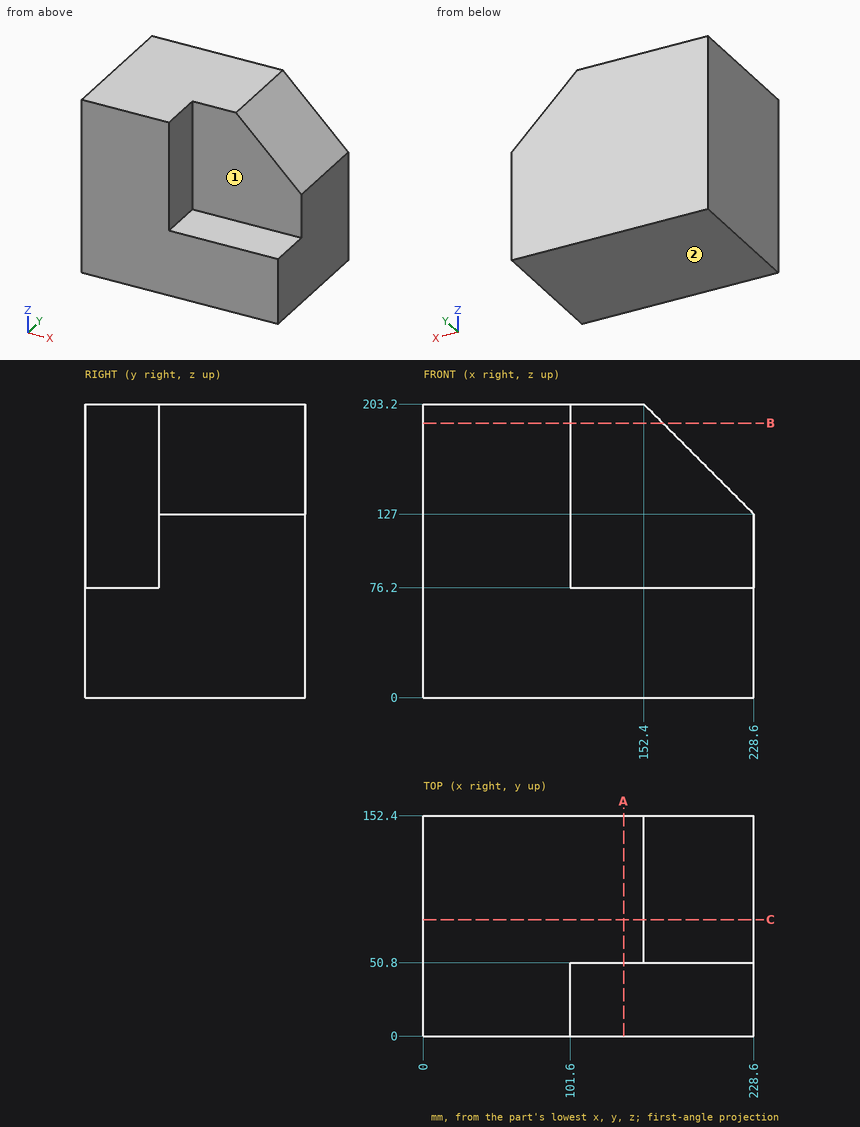
Source: three-view drawing plus pictorial views. Frame: mm from the lowest corner of the part. A direction names the side the tool comes from. Coordinates: 2 decimals unless noted, no trailing zeros. Order: outer loops, then holes, each group sorted by start corner. A loop starts at its lowest first (then second) coordinate and runs counter-clockwise, first axis right, second up. Notation, with made-up numbers: (39, 61.25) -> (70, 61.25) arc R22 ccw to (70, 70.25) -> close; hole circle Ø5 at (-23.75, 0.5). An arc over 180 degrees is marked (long way). Write item = value, one per line.
(1) Cut plane B-B on z = 190. Return loops of the section in (x, y), plus the area to 3 significant figures.
Solved:
outline = (0, 0) -> (101.6, 0) -> (101.6, 50.8) -> (165.6, 50.8) -> (165.6, 152.4) -> (0, 152.4) -> close
area = 22,000 mm²
(2) Line query: line 1 (Z direction, x = 190.5, y = 46); line 2 (Y direction, x = 163, z = 125); line 3 (X direction, y = 50, z = 114.5). Output: solid intervals per line, ascending.
Solved:
line_1 = 0 to 76.2
line_2 = 50.8 to 152.4
line_3 = 0 to 101.6
(3) Cut plane A-A on x = 138.5. Return loops of the section in (y, z), plus the area to 3 significant figures.
Solved:
outline = (0, 0) -> (152.4, 0) -> (152.4, 203.2) -> (50.8, 203.2) -> (50.8, 76.2) -> (0, 76.2) -> close
area = 24,500 mm²
(4) Access query for the marked faces 1 and 2. Directions: +Z, -Z, +X, -X, +Y, -Y. A direction counts if a zero-diameter tool reaches every point of the face in a straight line with its end or side. Return the directions, or none.
Solved:
face_1 = +Z, +X, -Y
face_2 = -Z, +X, -X, +Y, -Y
(5) Cut plane C-C on y = 80.5. Return loops of the section in (x, z).
Solved:
outline = (0, 0) -> (228.6, 0) -> (228.6, 127) -> (152.4, 203.2) -> (0, 203.2) -> close
(6) Pin query (flat end, axial travel): pin 1 Ø1 at (x, z) = (176, 106) entering from -Y; pin 2 Ø4 at (x, y) = (176, 104.5) entering from +Z. Return the tip coordinate at first contact, or that it passes through.
Solved:
pin_1 = 50.8
pin_2 = 181.6
